Study the drawing (mm; zero at the part's minimum x, y, z) and answer. A direction names the side the tool comes from. Round coordinates to 2 decimals unless told otherwise and drop trailing zeros. Loops run counter-clockwise (first coordinate to the right, second up) from the corner with the lowest first, then second, coordinate; pieces in that order, holes last. Notation, with made-up numbers: (49.5, -11) - (77.5, -11) arc R10 ccw to (77.5, -7) - close; hole circle Ø6 at (67, 82). An arc over 180 degrees is marked (long way). One line per item, written item: value.
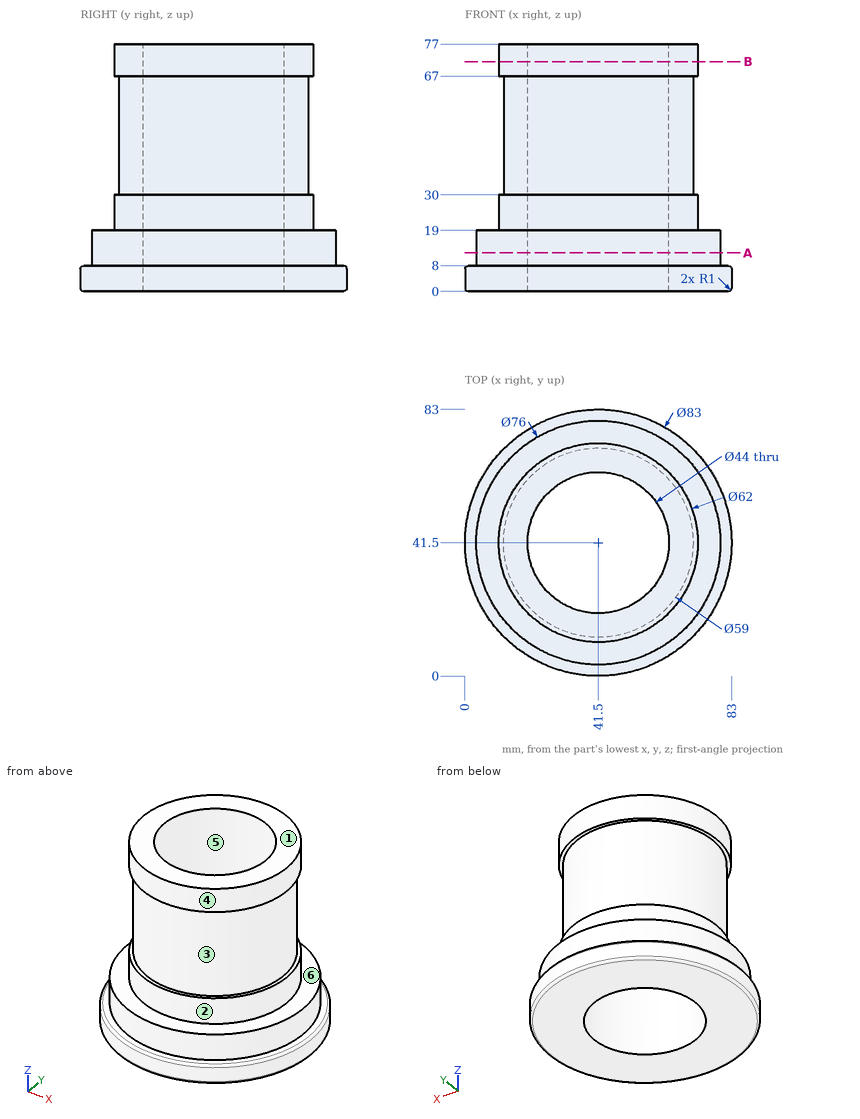
1) A cutting plane is placed at B-B on z = 71.5. Give the vertices of the cut face in (x, y), and give its area (3 significant figures).
Final values:
outline: circle Ø62 at (41.5, 41.5); hole circle Ø44 at (41.5, 41.5)
area: 1,500 mm2
2) Consider L1, parallel to Y at x = 41.5, z = 33.5; L2, parallel to Y at x = 41, z = 27; L3, parallel to Z at x = 59.5, y = 71. Determine where each line is inside the solid, lowest interval first.
Final values:
L1: 12 to 19.5, 63.5 to 71
L2: 10.5 to 19.51, 63.49 to 72.5
L3: 0 to 19
3) For a pull along X with two mould halves and no side action, classify the marked faces 4, 5 and 6 as released by +X, released by -X, zero draft, split by the parting line, or undercut.
Final values:
face 4: split by the parting line
face 5: undercut
face 6: zero draft
4) Each of these flat-tipped pins is pushed along its axis until it touches: pin 1 Ø5 at (x, z) = (17.5, 20) entering from -Y; pin 2 Ø6 at (x, y) = (56.5, 33.5) entering from -Z; pin 3 Ø4 at (x, z) = (17.5, 8.5) entering from -Y; pin 4 Ø1.5 at (y, z) = (68, 35) entering from +X. Where does it stop, or does it pass through?
Final values:
pin 1: y = 10.31
pin 2: through
pin 3: y = 6.62
pin 4: x = 55.89
5) For the marked faces 1, 2 and 3, determine the directions among +Z, -Z, +X, -X, +Y, -Y from which every point of the face is accessible in a straight line to the end or side of a thin tool.
Final values:
face 1: +Z, +X, -X, +Y, -Y
face 2: +Z
face 3: none
6) A cutting plane is placed at A-A on z = 12. Give the vertices of the cut face in (x, y).
Final values:
outline: circle Ø76 at (41.5, 41.5); hole circle Ø44 at (41.5, 41.5)
